```python
from build123d import *

# Parameters (mm, degrees)
SKETCH1_W           = 30
SKETCH1_H           = 55
BOSS_EXTRUDE1_DEPTH = 80
SKETCH2_W           = 70
SKETCH2_H           = 50
CUT_EXTRUDE1_DEPTH  = 60
SKETCH3_R           = 3.5
CUT_EXTRUDE2_DEPTH  = 117
SKETCH4_R           = 2.5
CUT_EXTRUDE3_DEPTH  = 42


with BuildPart() as part:
    # Sketch1 → Boss-Extrude1 (new body)
    with BuildSketch(Plane.XY):
        Rectangle(SKETCH1_W, SKETCH1_H)
    extrude(amount=BOSS_EXTRUDE1_DEPTH)

    # Sketch2 → Cut-Extrude1 (cut)
    with BuildSketch(Plane(origin=(15, 0, 0), x_dir=(0, 0, -1), z_dir=(1, 0, 0))):
        with Locations((-40, -2.5)):
            Rectangle(SKETCH2_W, SKETCH2_H)
    extrude(amount=-CUT_EXTRUDE1_DEPTH, mode=Mode.SUBTRACT)

    # Sketch3 → Cut-Extrude2 (cut)
    with BuildSketch(Plane.XY.offset(80)):
        with Locations((0, -12.5)):
            Circle(SKETCH3_R)
    extrude(amount=-CUT_EXTRUDE2_DEPTH, mode=Mode.SUBTRACT)

    # Sketch4 → Cut-Extrude3 (cut)
    with BuildSketch(Plane(origin=(0, 0, 0), x_dir=(1, 0, 0), z_dir=(0, 1, 0))):
        with Locations((0, -20)):
            Circle(SKETCH4_R)
        with Locations((0, -60)):
            Circle(SKETCH4_R)
    extrude(amount=CUT_EXTRUDE3_DEPTH, mode=Mode.SUBTRACT)


solid = part.part
```
Geometry: final body of the model. Coordinates: model frame, mm. A direction names the side the tool comes from. Round coordinates to 2 decimals unless told otherwise and drop trailing zeros. Write each loop counter-clockwise with the first axis right and the second up, starting at its lowest first coordinate (ties: lowest second). Pieces come first, ordered by that corner, then holes.
Item 1: Pin query (flat end, axial travel): P1, Ø2, axis at x = -1, z = 35, coming from the -Y side; P2, Ø4, axis at x = 0, y = -12.5, coming from the +Z side. Return the tip coordinate at first contact, or that it passes through.
Item 2: Mould query, pull axis X, two halves, no side actions, for faces 1 (the face through (1.34, 24.96, 57.89)), 2 (the face through (-15, 24, 46)), 3 (the face through (0, -3, 75)). Classes: +X half, -X half, draft (parallel to the pull), parting line (faces both ways), or undercut.
Item 3: Section query A-A (y = 18). Return loops of the section in (x, z), plus the area to 3 significant figures.
Item 4: Section query D-D (y = -12.5). Return loops of the section in (x, z).
Item 5: Section query C-C (z = 20). Return loops of the section in (x, y), plus the area to 3 significant figures.
Item 6: Material intervals for L1, parallel to Z at x = 0, y = 26.2; L2, parallel to Z at x = -2, y = 2; L3, parallel to Y at x = -6.25, z = 44.5, sorted ascending.
Item 7: Set-up query: faces 4 (the face through (0, 22.5, 40)), 5 (the face through (1.34, 24.96, 17.89)). Return all of +Z, -Z, +X, -X, +Y, -Y with unobstructed straight access to the full face (end or side cutting, diameter ignored); none if empty.
Item 8: Section query B-B (x = 0). Return loops of the section in (y, z).
Completed:
1. P1: stops at y = 22.5
1. P2: passes through
2. face 1: undercut
2. face 2: -X half
2. face 3: draft
3. outline: (-15, 0) - (15, 0) - (15, 5) - (-15, 5) - close; (-15, 75) - (15, 75) - (15, 80) - (-15, 80) - close
3. area: 300 mm2
4. outline: (-15, 0) - (-3.5, 0) - (-3.5, 5) - (-15, 5) - close; (-15, 75) - (-3.5, 75) - (-3.5, 80) - (-15, 80) - close; (3.5, 0) - (15, 0) - (15, 5) - (3.5, 5) - close; (3.5, 75) - (15, 75) - (15, 80) - (3.5, 80) - close
5. outline: (-15, 22.5) - (-2.5, 22.5) - (-2.5, 27.5) - (-15, 27.5) - close; (2.5, 22.5) - (15, 22.5) - (15, 27.5) - (2.5, 27.5) - close
5. area: 125 mm2
6. L1: z = 0 to 17.5, 22.5 to 57.5, 62.5 to 80
6. L2: z = 0 to 5, 75 to 80
6. L3: y = 22.5 to 27.5
7. face 4: +X, -X, -Y
7. face 5: +Y, -Y
8. outline: (-27.5, 0) - (-16, 0) - (-16, 5) - (-27.5, 5) - close; (-27.5, 75) - (-16, 75) - (-16, 80) - (-27.5, 80) - close; (-9, 0) - (27.5, 0) - (27.5, 17.5) - (22.5, 17.5) - (22.5, 5) - (-9, 5) - close; (-9, 75) - (22.5, 75) - (22.5, 62.5) - (27.5, 62.5) - (27.5, 80) - (-9, 80) - close; (22.5, 22.5) - (27.5, 22.5) - (27.5, 57.5) - (22.5, 57.5) - close
